Geometry: final body of the model. Coordinates: model frame, mm. A direction names the side the tool comes from. Give positions to 0.01 mm unless a question says otherwise; leave off trailing zeros. Order: outer loops, then holes, each group sorted by start corner. A loop starts at its lowest first (then second) coordinate and runs counter-clockwise, first axis right, second up. Notation, with made-up numbers: (-9, -36.75) -> (31, -36.75) arc R16 ccw to (31, -6.75) -> close; hole circle Ø6 at (34, 33.25). An arc over 180 degrees is marked (long way). Write item = value, one per line.
```python
from build123d import *

# Parameters (mm, degrees)
F2_R      = 17.075
F0_R      = 15.1
F5_R      = 10.75
F5_R_2    = 10
F6_DEPTH  = 18
F7_DEPTH  = 18
F8_R      = 10
F8_R_2    = 7.45
F9_DEPTH  = 2
F11_DEPTH = 3.8


with BuildPart() as f3:
    # F2 (on offset) → F3 section 0
    with BuildSketch(Plane.XY.offset(-12.7)):
        Circle(F2_R)
    # F0 (on Top) → F3 section 1
    with BuildSketch(Plane.XY):
        Circle(F0_R)
    loft()

    # F5 (on offset) → F6 (join)
    with BuildSketch(Plane.XY.offset(-18)):
        Circle(F5_R)
        Circle(F5_R_2, mode=Mode.SUBTRACT)
    extrude(amount=F6_DEPTH)

    # F7 (cut): a face of the model
    f7_faces = [f3.faces().sort_by_distance(p)[0] for p in [
        (0, 0, -12.7),
    ]]
    extrude(f7_faces, amount=-F7_DEPTH, mode=Mode.SUBTRACT)

    # F8 (on Top) → F9 (join)
    with BuildSketch(Plane.XY):
        Circle(F8_R)
        Circle(F8_R_2, mode=Mode.SUBTRACT)
    extrude(amount=-F9_DEPTH)

    # F10 (on face) → F11 (join)
    with BuildSketch(Plane(origin=(0, 0, -18), x_dir=(1, 0, 0), z_dir=(0, 0, -1))):
        with BuildLine():
            Line((-14.05, 2.5), (-14.05, 0))
            Line((-14.05, 0), (-14.05, -2.5))
            Line((-14.05, -2.5), (-10.4552618332, -2.5))
            ThreePointArc((-10.4552618332, -2.5), (-10.75, 0), (-10.4552618332, 2.5))
            Line((-10.4552618332, 2.5), (-14.05, 2.5))
        make_face()
        with BuildLine():
            Line((14.05, 2.5), (10.4552618332, 2.5))
            ThreePointArc((10.4552618332, 2.5), (10.6760611816, 1.2586570807), (10.75, 0))
            ThreePointArc((10.75, 0), (10.6760611816, -1.2586570807), (10.4552618332, -2.5))
            Line((10.4552618332, -2.5), (14.05, -2.5))
            Line((14.05, -2.5), (14.05, 0))
            Line((14.05, 0), (14.05, 2.5))
        make_face()
    extrude(amount=-F11_DEPTH)


solid = f3.part
```
1) Mould query, pull axis X, two halves, no side actions, for faces 5 (the face through (12, 0, -14.2)), 6 (the face through (7.106, 2.238, -0.986)), 7 (the face through (10.254, 3.229, -15.387)), 8 (the face through (14.05, 0, -16)). Classes: +X half, -X half, draft (parallel to the pull), parting line (faces both ways), or undercut.
Check sheet entries:
face_5 = draft
face_6 = undercut
face_7 = parting line
face_8 = +X half
2) Section query C-C (z = -3). Output: boundary loops of the cut face in (x, y), plus the area to 3 significant figures.
Check sheet entries:
outline = circle Ø31.13 at (0, 0); hole circle Ø20 at (0, 0)
area = 447 mm²
3) First-contact query: P1, Ø4, axis at x = -13, z = -17, coming from the -Y side; P2, Ø1, axis at y = -11.5, z = -8, coming from the +X side; P3, Ø1.1, axis at y = 1, z = -16.5, coming from the -X side. Flat tips, straight axial feed; report the tip coordinate or a pass-through.
Check sheet entries:
P1 = -2.5
P2 = 12.1
P3 = -14.05
4) Section query A-A (x = 0). Output: boundary loops of the cut face in (y, z) (3 decimals).
Check sheet entries:
outline = (-17.075, -12.7) -> (-10.75, -12.7) -> (-10.75, -18) -> (-10, -18) -> (-10, -2) -> (-7.45, -2) -> (-7.45, 0) -> (-15.1, 0) -> close; (7.45, -2) -> (10, -2) -> (10, -18) -> (10.75, -18) -> (10.75, -12.7) -> (17.075, -12.7) -> (15.1, 0) -> (7.45, 0) -> close
5) Line query: line 1 (X direction, y = 0, z = -15.3); line 2 (Y direction, x = 0, z = -14.75). Output: solid intervals per line, ascending. Write a range as from..to.
Check sheet entries:
line_1 = -14.05..-10, 10..14.05
line_2 = -10.75..-10, 10..10.75
6) Reachability of faces 1 (the face through (-12, 2.5, -16)), 2 (the face through (12, -2.5, -16)), 3 (the face through (-14.05, 0, -16)), 4 (the face through (12, 2.5, -16)) from +Z, -Z, +X, -X, +Y, -Y: full face, straight path, thin tool, end or side. Return the list, or none.
Check sheet entries:
face_1 = -Z, -X, +Y
face_2 = -Z, +X, -Y
face_3 = -Z, -X, +Y, -Y
face_4 = -Z, +X, +Y
7) Section query B-B (z = -15). Output: boundary loops of the cut face in (x, y).
Check sheet entries:
outline = (-14.05, -2.5) -> (-10.46, -2.5) arc R10.75 ccw to (10.46, -2.5) -> (14.05, -2.5) -> (14.05, 2.5) -> (10.46, 2.5) arc R10.75 ccw to (-10.46, 2.5) -> (-14.05, 2.5) -> close; hole circle Ø20 at (0, 0)
